```python
from build123d import *

# Parameters (mm, degrees)
BOSS_EXTRUDE1_DEPTH = 100


with BuildPart() as part:
    # Sketch1 → Boss-Extrude1 (new body)
    with BuildSketch(Plane.XY):
        Polygon((-42.640501462, 0), (0, 0), (0, 1.805938608), (-41.76781617, 1.805938608), (-41.76781617, 2.603006823), (-44.734392464, 2.603006823), (-44.734392464, 6.522673981), (-46.8, 6.522673981), (-46.8, 8.122673981), (-44.7, 10.188281516), (-44.7, 37.494976181), (-46.8, 37.494976181), (-46.8, 39.094976181), (-44.767698794, 39.094976181), (-44.767698794, 41.705938608), (-24.973882416, 41.705938608), (-24.973882416, 43.24560851), (0, 43.24560851), (0, 45.023153475), (-21.988241511, 44.824503247), (-21.988241511, 45.21521639), (-47.498865937, 45.21521639), (-48.3, 44.427202791), (-48.3, 1.384902814), (-48.656798132, 1.033948095), (-57.3, 1.033948095), (-57.3, -1.08478361), (-43.743346771, -1.08478361), align=None)
        Polygon((0, 0), (42.640501462, 0), (43.743346771, -1.08478361), (57.3, -1.08478361), (57.3, 1.033948095), (48.656798132, 1.033948095), (48.3, 1.384902814), (48.3, 44.427202791), (47.498865937, 45.21521639), (21.988241511, 45.21521639), (21.988241511, 44.824503247), (0, 45.023153475), (0, 43.24560851), (24.973882416, 43.24560851), (24.973882416, 41.705938608), (44.767698794, 41.705938608), (44.767698794, 39.094976181), (46.8, 39.094976181), (46.8, 37.494976181), (44.7, 37.494976181), (44.7, 10.188281516), (46.8, 8.122673981), (46.8, 6.522673981), (44.734392464, 6.522673981), (44.734392464, 2.603006823), (41.76781617, 2.603006823), (41.76781617, 1.805938608), (0, 1.805938608), align=None)
    extrude(amount=BOSS_EXTRUDE1_DEPTH)


solid = part.part
```
CAD build for the part. Positions are in the model's coordinates, mm. A direction names the side the tool comes from. Give positions to 0.01 mm unless a question says otherwise; leave off trailing zeros. Loops run counter-clockwise (first coordinate to the right, second up) from the corner with the lowest first, then second, coordinate; pieces in that order, holes last. Notation, with made-up numbers: (72, 64.25) - (91, 64.25) arc R31 cw to (91, 92.25) - close; hole circle Ø5 at (-33, -14). An arc over 180 degrees is marked (long way). Put each result on its own line as item: value.
Q1. Mould opens along Y. For faces 1 (the face through (-44.7, 24, 49)), 2 (the face through (-53, 1.034, 49)), 3 (the face through (-1, 0, 49)) say: pulls with the +Y half, pulls with the -Y half, needs draft (parallel to the pull), parting line crosses it, or undercut.
Filled in:
face 1: undercut
face 2: pulls with the +Y half
face 3: pulls with the -Y half
Q2. Slice it at A-A (x = -38). Give the cut face in (y, z).
Filled in:
outline: (0, 0) - (1.81, 0) - (1.81, 100) - (0, 100) - close; (41.71, 0) - (45.22, 0) - (45.22, 100) - (41.71, 100) - close
Q3. Tool access for faces 4 (the face through (53, 1.034, 49)), 5 (the face through (50, -1.085, 49)), 6 (the face through (0, 43.246, 49)): list every direction of +Z, -Z, +X, -X, +Y, -Y with a clear straight run to the whole face (end or side of a thin tool).
Filled in:
face 4: +Z, -Z, +X, +Y
face 5: +Z, -Z, +X, -X, -Y
face 6: +Z, -Z
Q4. Probe line 1 along Y through (x, z) = (-2, 9); line 2 along X through (y, z) = (22, 6); line 3 along Y through (x, z) = (-40, 48). List the from-to ranges inside material, lowest first.
Filled in:
line 1: y = 0 to 1.81, 43.25 to 45.01
line 2: x = -48.3 to -44.7, 44.7 to 48.3
line 3: y = 0 to 1.81, 41.71 to 45.22
Q5. Flat gauge pins, fed straight in: pin 1 (4 mm diameter, centred on y = 13, z = 70.5, fed in from +X); pin 2 (4 mm diameter, centred on y = 11.5, z = 58.5, fed in from -X); pin 3 (1 mm diameter, centred on x = 21, z = 70.5, fed in from +Y). Where does each tip first touch, or does it go through?
Filled in:
pin 1: stops at x = 48.3
pin 2: stops at x = -48.3
pin 3: stops at y = 44.84
Q6. Slice it at B-B (y = 4). Give the cut face in (x, z), plus the area to 3 significant figures.
Filled in:
outline: (-48.3, 0) - (-44.73, 0) - (-44.73, 100) - (-48.3, 100) - close; (44.73, 0) - (48.3, 0) - (48.3, 100) - (44.73, 100) - close
area: 713 mm²
